Verification items for the finished model (mm, model axes). Face numbers are marked on the shaded views. A direction names the side the tool comes from. Give positions to 0.01 mm unless a question says otherwise; leave off trailing zeros. Loops run counter-clockwise (first coordinate to the right, second up) from the corner with the lowest first, then second, coordinate; pieces in that order, holes last. Notation, with made-up numbers: M -26,-25.75 L 17,-25.75 A25 cw 17,5.25 Z; hole C -34.75,38 d11. An arc over 180 degrees is marked long. Use a Markdown table: item, result.
from build123d import *

# Parameters (mm, degrees)
BOSS_EXTRUDE1_DEPTH = 18
SKETCH2_W           = 68
SKETCH2_H           = 20
CUT_EXTRUDE2_DEPTH  = 2
SKETCH4_W           = 20
SKETCH4_H           = 20
CUT_EXTRUDE3_DEPTH  = 7
SKETCH5_R           = 6.163168956
CUT_EXTRUDE4_DEPTH  = 103.004901843
CUT_EXTRUDE5_START  = -41
CUT_EXTRUDE5_DEPTH  = 41
FILLET1_R           = 6


with BuildPart() as part:
    # Sketch1 → Boss-Extrude1 (new, symmetric)
    with BuildSketch(Plane.XY):
        with BuildLine():
            Line((-84, 0), (84, 0))
            Line((84, 0), (80, 14))
            Line((80, 14), (43, 14))
            Line((43, 14), (43, 55))
            Line((43, 55), (22, 55))
            Line((22, 55), (22, 43))
            Line((22, 43), (19, 43))
            Line((19, 43), (19, 40))
            ThreePointArc((19, 40), (0, 21), (-19, 40))
            Line((-19, 40), (-19, 43))
            Line((-19, 43), (-22, 43))
            Line((-22, 43), (-22, 55))
            Line((-22, 55), (-43, 55))
            Line((-43, 55), (-43, 14))
            Line((-43, 14), (-80, 14))
            Line((-80, 14), (-84, 0))
        make_face()
    extrude(amount=BOSS_EXTRUDE1_DEPTH, both=True)

    # Sketch2 → Cut-Extrude2 (cut)
    with BuildSketch(Plane.XZ):
        with Locations((-42, 0)):
            Rectangle(SKETCH2_W, SKETCH2_H)
        with Locations((42, 0)):
            Rectangle(SKETCH2_W, SKETCH2_H)
    extrude(amount=-CUT_EXTRUDE2_DEPTH, mode=Mode.SUBTRACT)

    # Sketch4 → Cut-Extrude3 (cut)
    with BuildSketch(Plane.XZ.offset(-2)):
        with Locations((-31, 0)):
            Rectangle(SKETCH4_W, SKETCH4_H)
        with Locations((31, 0)):
            Rectangle(SKETCH4_W, SKETCH4_H)
    extrude(amount=-CUT_EXTRUDE3_DEPTH, mode=Mode.SUBTRACT)

    # Sketch5 → Cut-Extrude4 (cut, through all)
    with BuildSketch(Plane.XZ):
        with Locations((-31, 0)):
            Circle(SKETCH5_R)
        with Locations(Location((31, 0, 0), (0, 0, 180))):
            Circle(SKETCH5_R)
        with BuildLine():
            Line((-68, 5), (-60, 5))
            ThreePointArc((-60, 5), (-55, 0), (-60, -5))
            Line((-60, -5), (-68, -5))
            ThreePointArc((-68, -5), (-73, 0), (-68, 5))
        make_face()
        with BuildLine():
            Line((68, 5), (60, 5))
            ThreePointArc((60, 5), (55, 0), (60, -5))
            Line((60, -5), (68, -5))
            ThreePointArc((68, -5), (73, 0), (68, 5))
        make_face()
    extrude(amount=-CUT_EXTRUDE4_DEPTH, mode=Mode.SUBTRACT)

    # Cut-Extrude5: read off the stored shape, not the designer's step
    # Cut-Extrude5 outline → Cut-Extrude5 (cut)
    with BuildSketch(Plane(origin=(0, 55, 0), x_dir=(1, 0, 0), z_dir=(0, 1, 0)).offset(CUT_EXTRUDE5_START)):
        with BuildLine():
            ThreePointArc((-43, 0), (-42.001212365, 9.214019744), (-39.05124838, 18))
            Line((-39.05124838, 18), (-43, 18))
            Line((-43, 18), (-43, 0))
        make_face()
        with BuildLine():
            ThreePointArc((-39.05124838, -18), (-42.001212365, -9.214019744), (-43, 0))
            Line((-43, 0), (-43, -18))
            Line((-43, -18), (-39.05124838, -18))
        make_face()
        with BuildLine():
            Line((43, 18), (39.05124838, 18))
            ThreePointArc((39.05124838, 18), (42.001212365, 9.214019744), (43, 0))
            Line((43, 0), (43, 18))
        make_face()
        with BuildLine():
            Line((43, -18), (43, 0))
            ThreePointArc((43, 0), (42.001212365, -9.214019744), (39.05124838, -18))
            Line((39.05124838, -18), (43, -18))
        make_face()
    extrude(amount=CUT_EXTRUDE5_DEPTH, mode=Mode.SUBTRACT)

    # Fillet1
    fillet1_edges = [part.edges().sort_by_distance(p)[0] for p in [
        (-42.001212365, 14, 9.214019744),
        (42.001212365, 14, -9.214019744),
    ]]
    fillet(fillet1_edges, radius=FILLET1_R)

    # Cut-Revolve1: read off the stored shape, not the designer's step
    # Cut-Revolve1 outline → Cut-Revolve1 (revolve, cut)
    with BuildSketch(Plane.XY):
        Polygon((0, 13.435755104), (3, 15.238336961), (3, 21.238467133), (0, 21.238467133), align=None)
    revolve(axis=Axis((0, 0, 0), (0, 1, 0)), mode=Mode.SUBTRACT)


solid = part.part
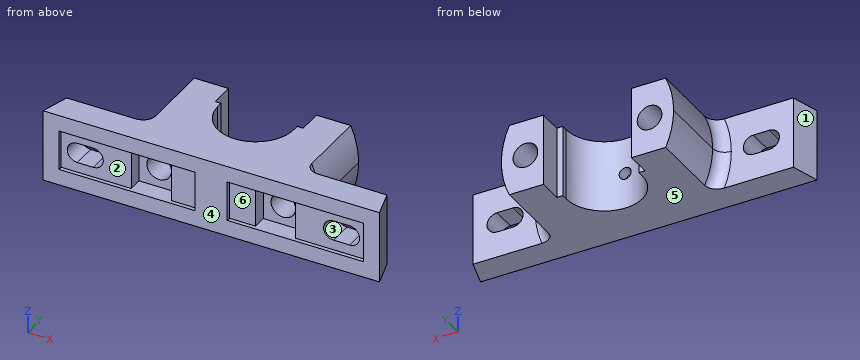
(1) Cross-section at D-D on y = 7.5. Record the cut outline in (x, z).
Results below:
| item | result |
|---|---|
| outline | M -81.86,-18 L 81.86,-18 L 81.86,18 L -81.86,18 Z; hole M -68,-5 L -60,-5 A5 ccw -60,5 L -68,5 A5 ccw Z; hole M -41,-10 L -21,-10 L -21,10 L -41,10 Z; hole M 21,-10 L 41,-10 L 41,10 L 21,10 Z; hole M 60,-5 L 68,-5 A5 ccw 68,5 L 60,5 A5 ccw Z |
(2) Gauge pin test, flat ends, axial feed: P1, Ø1, axis at x = -45, y = 49, coming from the +Z side; P2, Ø7.5, axis at y = 7, z = -1.5, coming from the -X side; P3, Ø1.5, axis at x = 57.5, z = 6.5, coming from the -Y side; P4, Ø0.6, axis at y = 1, z = 3, coming from the +X side. Record the tip position at first contact, or that the pin passes through.
Results below:
| item | result |
|---|---|
| P1 | through |
| P2 | x = -83.07 |
| P3 | y = 2 |
| P4 | x = 83.8 |
(3) Cross-section at C-C on x = 51. Record the cut outline in (y, z).
Results below:
| item | result |
|---|---|
| outline | M 0,-18 L 14,-18 L 14,18 L 0,18 L 0,10 L 2,10 L 2,-10 L 0,-10 Z |
(4) Material ranges on line 1 (X direction, y = 22.5, z = -1); line 2 (Z direction, x = 0, y = 17); line 3 (X direction, y = 49.5, z = -3.5), recorded low to high.
Results below:
| item | result |
|---|---|
| line 1 | -42.99 to -37.08, -24.92 to -7.4, 7.4 to 24.92, 37.08 to 42.99 |
| line 2 | -18 to -3, 3 to 18 |
| line 3 | -42.86 to -36.07, -25.93 to -22, 22 to 25.93, 36.07 to 42.86 |
(5) Cross-section at A-A on x = -31. Record the cut outline in (y, z).
Results below:
| item | result |
|---|---|
| outline | M 0,-18 L 55,-18 L 55,-6.16 L 9,-6.16 L 9,-10 L 0,-10 Z; M 0,10 L 9,10 L 9,6.16 L 55,6.16 L 55,18 L 0,18 Z |
(6) Cross-section at B-B on y = 36. Record the cut outline in (x, z), then the cut area to 3 significant figures.
Results below:
| item | result |
|---|---|
| outline | M -39.05,-18 L -18.57,-18 L -18.57,18 L -39.05,18 A43 ccw Z; M 18.57,-18 L 39.05,-18 A43 ccw 39.05,18 L 18.57,18 Z; hole C -31,0 d12.33; hole C 31,0 d12.33 |
| area | 1,430 mm^2 |
(7) Draft check along Z on the marked faces 4, 5 and 6. Enter one of: +Z half, -Z half, draft (parallel to the pull), parting line (faces both ways), or undercut.
Results below:
| item | result |
|---|---|
| face 4 | draft |
| face 5 | -Z half |
| face 6 | undercut |
(8) Set-up check for the marked faces 1, 2 and 3: record each of +Z, -Z, +X, -X, +Y, -Y from which the full face is reachable in a straight line by a thin tool's end or side.
Results below:
| item | result |
|---|---|
| face 1 | +Z, -Z, -X, +Y |
| face 2 | -Y |
| face 3 | +Y, -Y |
